Model file for the job. Use its own axes, mm. Face numbers are marked on the shaded views. Coordinates: 2 decimals unless noted, no trailing zeros. Order: outer loops, then holes, each group sorted by start corner. A loop starts at its lowest first (then second) coordinate and runs counter-clockwise, first axis right, second up. Notation, with made-up numbers: M 26.5,83.5 L 66.5,83.5 A26 cw 66.5,122.5 Z; hole C 44,-2 d1. An arc over 180 degrees is marked long. Return JSON: item names as keys, results as strings.
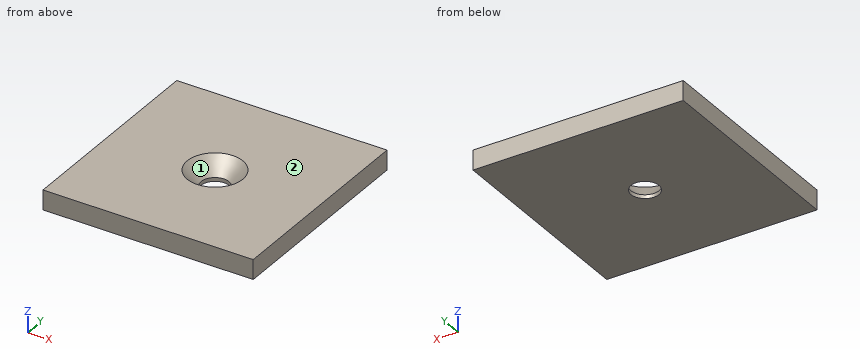
```python
from build123d import *

# Parameters (mm, degrees)
SKETCH1_W           = 50.8
SKETCH1_H           = 50.8
BOSS_EXTRUDE1_DEPTH = 4.7625


with BuildPart() as part:
    # Sketch1 → Boss-Extrude1 (new body)
    with BuildSketch(Plane.XY):
        with Locations((25.4, -25.4)):
            Rectangle(SKETCH1_W, SKETCH1_H)
    extrude(amount=BOSS_EXTRUDE1_DEPTH)

    # Sketch4 → CSK for 1/4 Flat Head Machine Screw (100)1 (revolve, cut)
    with BuildSketch(Plane(origin=(25.4, -25.4, 4.7625), x_dir=(0, -1, 0), z_dir=(1, 0, 0))):
        Polygon((0, 0), (0, 4.7625), (3.3782, 4.7625), (3.3782, 3.856955196), (6.731, 0), align=None)
    revolve(axis=Axis((25.4, -25.4, 11.1125), (0, 0, -1)), mode=Mode.SUBTRACT)


solid = part.part
```
Item 1: Drop flat-ended pins along their axis: pin 1 Ø1.5 at (x, z) = (45, 2.5) entering from +Y; pin 2 Ø8 at (x, y) = (25.4, -25.4) entering from +Z. Give the stop position or say it passes through.
Check result:
{"pin 1": "stops at y = 0", "pin 2": "stops at z = 1.62"}
Item 2: Saw through at B-B (x = 25.4). Write the cut outline in (y, z).
Check result:
{"outline": "M -50.8,0 L -28.78,0 L -28.78,0.91 L -32.13,4.76 L -50.8,4.76 Z; M -22.02,0 L 0,0 L 0,4.76 L -18.67,4.76 L -22.02,0.91 Z"}
Item 3: Wall check: line 1 (X direction, y = -25.4, z = 0.4); line 2 (Y direction, x = 25.4, z = 0.4); line 3 (X direction, y = -22, z = 4.35). Give the ranges that are in metal, low to high.
Check result:
{"line 1": "x = 0 to 22.02, 28.78 to 50.8", "line 2": "y = -50.8 to -28.78, -22.02 to 0", "line 3": "x = 0 to 20.01, 30.79 to 50.8"}
Item 4: Saw through at A-A (y = -25.4). Write the cut outline in (x, z), and give its area (3 significant figures).
Check result:
{"outline": "M 0,0 L 22.02,0 L 22.02,0.91 L 18.67,4.76 L 0,4.76 Z; M 28.78,0 L 50.8,0 L 50.8,4.76 L 32.13,4.76 L 28.78,0.91 Z", "area": "197 mm2"}
Item 5: Pull direction X, two halves, no side cores. Call the marked faces 1 and 2: +X half, -X half, draft (parallel to the pull), parting line (faces both ways), or undercut.
Check result:
{"face 1": "undercut", "face 2": "draft"}
